Check sheet for the modelled part. Datum: model origin and axes. Units: mm. A direction names the side the tool comes from. Round coordinates to 2 decimals unless told otherwise and drop trailing zeros. Write each loop counter-clockwise with the first axis right and the second up, starting at its lowest first coordinate (ties: lowest second). Pieces come first, ordered by that corner, then holes.
Item 1: Material ranges on line 1 (X direction, y = 2.9, z = 3) (3 decimals); line 2 (Z direction, x = 0, y = 3.65); line 3 (X direction, y = -1.75, z = 3.75) (3 decimals), recorded low to high.
Item 2: Cross-section at A-A on x = 0. Enter the section's corners in (y, z).
Item 3: Go/stop test with flat-tipped pins: pin 1 Ø1.5 at (x, y) = (0, 0.5) entering from -Z; pin 2 Ø1.8 at (y, z) = (-3, 3) entering from +X (3 decimals); pin 3 Ø1.4 at (x, z) = (0, 3) entering from +Y; pin 4 Ø0.8 at (x, z) = (1, 2) entering from -Y. Record where each tip stops, or that it passes through.
Item 4: Cross-section at B-B on z = 3. Enter the section's corners in (x, y) (3 decimals), plus the area to 3 significant figures.
Item 5: Release check for a two-part mould opening along X. For faces 1 (the flat face through (-1.925, 0, 3)), 2 (the flat face through (0, 1, 3)), 3 (the flat face through (1, 6, 3)), 4 (the cylindrical face through (-0.52, 3.54, 2.33)) record: +X half, -X half, draft (parallel to the pull), parting line (faces both ways), or undercut.
Item 6: Cross-section at C-C on y = 1.5. Enter the section's corners in (x, z) (3 decimals).
Item 7: Cross-section at D-D on z = 4.9. Enter the section's corners in (x, y) (3 decimals), plus the area to 3 significant figures.
Item 8: Tool access check on faces 5 (the flat face through (1, 1, 3)), 6 (the flat face through (-1, -6, 3)). Record the directions out of +Z, -Z, +X, -X, +Y, -Y that give a thin tool (end or side, any length) a straight path to the whole face; none if there is none.
from build123d import *

# Parameters (mm, degrees)
BOSS_EXTRUDE1_DEPTH = 6
SKETCH2_R           = 0.85
CUT_EXTRUDE1_DEPTH  = 10.317859196
SKETCH3_R           = 0.85
CUT_EXTRUDE2_DEPTH  = 5


with BuildPart() as part:
    # Sketch1 → Boss-Extrude1 (new body)
    with BuildSketch(Plane.XY):
        Polygon((-1.925, -6), (0.425, -6), (0.425, 1), (1.925, 1), (1.925, 6), (-1.925, 6), align=None)
    extrude(amount=BOSS_EXTRUDE1_DEPTH)

    # Sketch2 → Cut-Extrude1 (cut, through all)
    with BuildSketch(Plane.ZY.offset(1.925)):
        with Locations(Location((3, -2.55134747, 0), (0, 0, 270))):
            Circle(SKETCH2_R)
    extrude(amount=-CUT_EXTRUDE1_DEPTH, mode=Mode.SUBTRACT)

    # Sketch3 → Cut-Extrude2 (cut)
    with BuildSketch(Plane(origin=(0, 6, 0), x_dir=(1, 0, 0), z_dir=(0, 1, 0))):
        with Locations(Location((0, -3, 0), (0, 0, 270))):
            Circle(SKETCH3_R)
    extrude(amount=-CUT_EXTRUDE2_DEPTH, mode=Mode.SUBTRACT)


solid = part.part
Response values:
1. line 1: x = -1.925 to -0.85, 0.85 to 1.925
1. line 2: z = 0 to 2.15, 3.85 to 6
1. line 3: x = -1.925 to 0.425
2. outline: (-6, 0) - (6, 0) - (6, 2.15) - (1, 2.15) - (1, 3.85) - (6, 3.85) - (6, 6) - (-6, 6) - close; hole circle Ø1.7 at (-2.55, 3)
3. pin 1: stops at z = 0
3. pin 2: stops at x = 0.425
3. pin 3: stops at y = 1
3. pin 4: stops at y = 1
4. outline: (-1.925, -6) - (0.425, -6) - (0.425, -3.401) - (-1.925, -3.401) - close; (-1.925, -1.701) - (0.425, -1.701) - (0.425, 1) - (-0.85, 1) - (-0.85, 6) - (-1.925, 6) - close; (0.85, 1) - (1.925, 1) - (1.925, 6) - (0.85, 6) - close
4. area: 23.2 mm2
5. face 1: -X half
5. face 2: undercut
5. face 3: draft
5. face 4: undercut
6. outline: (-1.925, 0) - (1.925, 0) - (1.925, 6) - (-1.925, 6) - close; hole circle Ø1.7 at (0, 3)
7. outline: (-1.925, -6) - (0.425, -6) - (0.425, 1) - (1.925, 1) - (1.925, 6) - (-1.925, 6) - close
7. area: 35.7 mm2
8. face 5: +Z, -Z, +X, -Y
8. face 6: +Z, -Z, +X, -X, -Y
